from build123d import *

# Parameters (mm, degrees)
ESQUISSE1_R        = 3
ESQUISSE1_R_2      = 1.5
BOSS_EXTRU_1_DEPTH = 5
CONG_1_R           = 6


with BuildPart() as part:
    # Esquisse1 → Boss.-Extru.1 (new body)
    with BuildSketch(Plane.XY):
        with BuildLine():
            Line((0, 8), (5, 8))
            Line((5, 8), (20, 5))
            Line((20, 5), (20, -8))
            Line((20, -8), (0, -8))
            ThreePointArc((0, -8), (-8, 0), (0, 8))
        make_face()
        Circle(ESQUISSE1_R, mode=Mode.SUBTRACT)
        with Locations((15, 0)):
            Circle(ESQUISSE1_R_2, mode=Mode.SUBTRACT)
    extrude(amount=BOSS_EXTRU_1_DEPTH)

    # Congé1
    cong_1_edges = [part.edges().sort_by_distance(p)[0] for p in [
        (20, 5, 2.5),
    ]]
    fillet(cong_1_edges, radius=CONG_1_R)


solid = part.part
Input: part model. Units: mm. Frame: model coordinates. Give positions to 0.01 mm unless a question says otherwise; leave off trailing zeros. Loops run counter-clockwise (first coordinate to the right, second up) from the corner with the lowest first, then second, coordinate; pieces in that order, holes last. Notation, with made-up numbers: (29.5, 43) -> (67.5, 43) arc R31 ccw to (67.5, 71) -> close; hole circle Ø5 at (56, 23). An arc over 180 degrees is marked (long way). Answer as a JSON object with one key per item and string values. Group by question number.
Item 1: Pin query (flat end, axial travel): P1, Ø5, axis at x = 0, y = 0, coming from the -Z side; P2, Ø3, axis at y = -5.5, z = 3.5, coming from the -X side; P3, Ø1, axis at y = -4, z = 4, coming from the -X side; P4, Ø1, axis at x = 9.5, z = 1, coming from the +Y side. Return the tip coordinate at first contact, or that it passes through.
Item 2: Cut plane B-B, the plane x = 0.75. Return the cut outline in (y, z), and give its area (3 significant figures).
Item 3: Line query: probe 1 along Y at (x, z) = (15, 0.7); probe 2 along X at (y, z) = (-2.25, 1.45); probe 3 along X at (y, z) = (2.75, 2.85). Output: solid intervals per line, ascending.
Item 4: Cut plane C-C, the plane x = 10.5. Return the cut outline in (y, z), and give its area (3 significant figures).
Item 5: Pull-direction query (Y, two-part tool) for faces 1 (the cylindrical face through (13.5, 0.07, 2.46)), 2 (the flat face through (2, 8, 2)), 3 (the flat face through (6, 0, 0)); classes: released by +Y, released by -Y, zero draft, split by the parting line, or undercut.
Item 6: Cut plane A-A, the plane z = 1.2. Return the cut outline in (x, y), and give its area (3 significant figures).
Item 7: Cut plane D-D, the plane y = -6.75. Return the cut outline in (x, z).
Checks:
{
 "1": {"P1": "passes through", "P2": "stops at x = -6.93", "P3": "stops at x = -7.19", "P4": "stops at y = 7.2"},
 "2": {"outline": "(-8, 0) -> (-2.9, 0) -> (-2.9, 5) -> (-8, 5) -> close; (2.9, 0) -> (8, 0) -> (8, 5) -> (2.9, 5) -> close", "area": "51.0 mm²"},
 "3": {"probe 1": "y = -8 to -1.5, 1.5 to 6", "probe 2": "x = -7.68 to -1.98, 1.98 to 20", "probe 3": "x = -7.51 to -1.2, 1.2 to 19.37"},
 "4": {"outline": "(-8, 0) -> (6.9, 0) -> (6.9, 5) -> (-8, 5) -> close", "area": "74.5 mm²"},
 "5": {"face 1": "undercut", "face 2": "released by +Y", "face 3": "zero draft"},
 "6": {"outline": "(0, -8) -> (20, -8) -> (20, 0.08) arc R6 ccw to (15.18, 5.96) -> (5, 8) -> (0, 8) arc R8 ccw to start; hole circle Ø6 at (0, 0); hole circle Ø3 at (15, 0)", "area": "358 mm²"},
 "7": {"outline": "(-4.29, 0) -> (20, 0) -> (20, 5) -> (-4.29, 5) -> close"}
}
